Geometry: see drawing. Coordinates: mm, zero at the bounding-box minimum. A direction names the side the tool comes from. Give positions to 0.01 mm unless a question says otherwise; leave off trailing zeros. Loops run counter-clockwise (first coordinate to the right, second up) from the corner with the lowest first, then second, coordinate; pieces in that order, holes last. Notation, with made-up numbers: (77, -26.75) -> (118, -26.75) arc R22 cw to (118, 6.25) -> close; hole circle Ø10 at (-26.75, 9). An arc over 180 degrees is marked (long way). One line per question, with ' | ' between items.
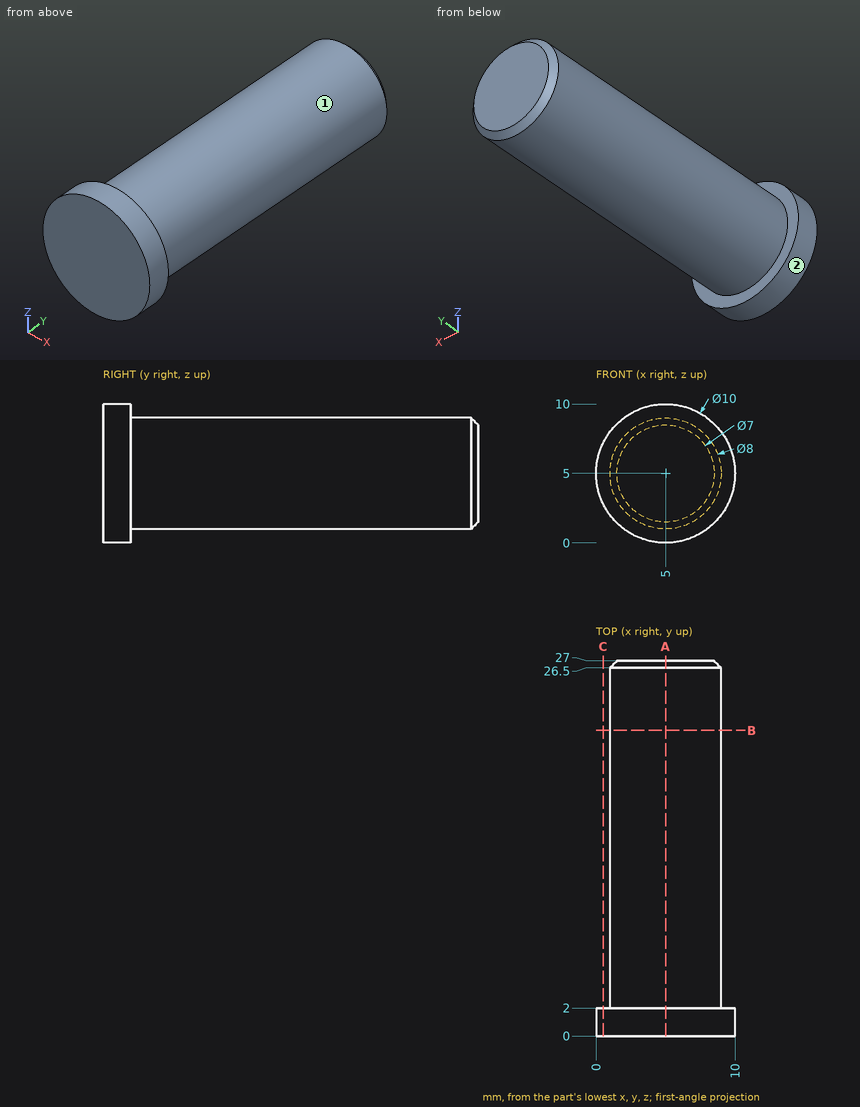
1. Reachability of the marked faces 1 and 2 from +Z, -Z, +X, -X, +Y, -Y: full face, straight path, thin tool, end or side. Return the list, or none.
Determined:
face 1: +Y | face 2: +Y, -Y
2. Section query C-C (x = 0.5). Output: boundary loops of the cut face in (y, z).
Determined:
outline: (0, 2.82) -> (2, 2.82) -> (2, 7.18) -> (0, 7.18) -> close
3. Pin query (flat end, axial travel): P1, Ø1, axis at x = 7, y = 24, coming from the +Z side; P2, Ø2, axis at y = 4.5, z = 6.5, coming from the +X side; P3, Ø1, axis at x = 5, y = 22, coming from the -Z side. Return the tip coordinate at first contact, or that it passes through.
Determined:
P1: stops at z = 8.71 | P2: stops at x = 8.97 | P3: stops at z = 1
4. Section query A-A (x = 5). Output: boundary loops of the cut face in (y, z), then the cut area to 3 significant figures.
Determined:
outline: (0, 0) -> (2, 0) -> (2, 1) -> (26.5, 1) -> (27, 1.5) -> (27, 8.5) -> (26.5, 9) -> (2, 9) -> (2, 10) -> (0, 10) -> close | area: 220 mm2
5. Section query B-B (y = 22). Output: boundary loops of the cut face in (x, z).
Determined:
outline: circle Ø8 at (5, 5)
6. Ray query, line 1 along Y through (x, z) = (2.5, 9.25); line 2 along Z through (x, y) = (6.5, 21.5); line 3 along X through (y, z) = (24.25, 4). Return the intervals inside material, ascending. Write a range as from..to.
Determined:
line 1: y = 0..2 | line 2: z = 1.29..8.71 | line 3: x = 1.13..8.87
